Can you work these out from the model? Positions are in its coordinate system, mm. A direction names the side the tool comes from. Coordinates: 2 decimals unless noted, no trailing zeros. Order: outer loops, then holes, each group sorted by start corner. A loop starts at its lowest first (then second) coordinate and runs counter-clockwise, first axis right, second up. Notation, with made-up numbers: (14.5, 24.5) -> (56.5, 24.5) arc R12 ccw to (56.5, 36.5) -> close; hole circle Ø2 at (-8.5, 72). An arc over 180 degrees is marked (long way). Answer as CSV lines item,"result".
from build123d import *

# Parameters (mm, degrees)
F0_R     = 25.527
F0_R_2   = 10.16
F1_DEPTH = 69.85
F0_R_3   = 26.797
F2_DEPTH = 1.27


with BuildPart() as f1:
    # F0 (on Top) → F1 (new body)
    with BuildSketch(Plane.XY):
        Circle(F0_R)
        with BuildLine():
            ThreePointArc((24.223731, 1.27), (24.248681, 0.635218), (24.257, 0))
            ThreePointArc((24.257, 0), (17.595574, -16.69724), (1.27, -24.223731))
            ThreePointArc((1.27, -24.223731), (0.635218, -24.248681), (0, -24.257))
            ThreePointArc((0, -24.257), (-17.152289, -17.152289), (-24.257, 0))
            ThreePointArc((-24.257, 0), (-24.248681, 0.635218), (-24.223731, 1.27))
            ThreePointArc((-24.223731, 1.27), (-16.69724, 17.595574), (0, 24.257))
            ThreePointArc((0, 24.257), (0.635218, 24.248681), (1.27, 24.223731))
            ThreePointArc((1.27, 24.223731), (17.152289, 17.152289), (24.223731, 1.27))
        make_face(mode=Mode.SUBTRACT)
        with BuildLine():
            ThreePointArc((1.27, -11.359225), (8.519419, -7.62), (11.43, 0))
            ThreePointArc((11.43, 0), (11.412293, 0.635985), (11.359225, 1.27))
            ThreePointArc((11.359225, 1.27), (8.082231, 8.082231), (1.27, 11.359225))
            ThreePointArc((1.27, 11.359225), (0.635985, 11.412293), (0, 11.43))
            ThreePointArc((0, 11.43), (-7.62, 8.519419), (-11.359225, 1.27))
            ThreePointArc((-11.359225, 1.27), (-11.412293, 0.635985), (-11.43, 0))
            ThreePointArc((-11.43, 0), (-8.082231, -8.082231), (0, -11.43))
            ThreePointArc((0, -11.43), (0.635985, -11.412293), (1.27, -11.359225))
        make_face()
        Circle(F0_R_2, mode=Mode.SUBTRACT)
        with BuildLine():
            Line((1.27, 11.359225), (1.27, 24.223731))
            ThreePointArc((1.27, 24.223731), (0.635218, 24.248681), (0, 24.257))
            Line((0, 24.257), (0, 11.43))
            ThreePointArc((0, 11.43), (0.635985, 11.412293), (1.27, 11.359225))
        make_face()
        with BuildLine():
            Line((11.43, 0), (24.257, 0))
            ThreePointArc((24.257, 0), (24.248681, 0.635218), (24.223731, 1.27))
            Line((24.223731, 1.27), (11.359225, 1.27))
            ThreePointArc((11.359225, 1.27), (11.412293, 0.635985), (11.43, 0))
        make_face()
        with BuildLine():
            ThreePointArc((0, -24.257), (0.635218, -24.248681), (1.27, -24.223731))
            Line((1.27, -24.223731), (1.27, -11.359225))
            ThreePointArc((1.27, -11.359225), (0.635985, -11.412293), (0, -11.43))
            Line((0, -11.43), (0, -24.257))
        make_face()
        with BuildLine():
            ThreePointArc((-24.223731, 1.27), (-24.248681, 0.635218), (-24.257, 0))
            Line((-24.257, 0), (-11.43, 0))
            ThreePointArc((-11.43, 0), (-11.412293, 0.635985), (-11.359225, 1.27))
            Line((-11.359225, 1.27), (-24.223731, 1.27))
        make_face()
    extrude(amount=F1_DEPTH)

    # F0 (on Top) → F2 (join)
    with BuildSketch(Plane.XY):
        Circle(F0_R_3)
        Circle(F0_R, mode=Mode.SUBTRACT)
    extrude(amount=F2_DEPTH)


solid = f1.part
Q1. Imagine slicing it at D-D (x = 8.5). List the corners of the cut face in (y, z) for me.
Solution:
outline,"(-25.41, 0) -> (-22.72, 0) -> (-22.72, 69.85) -> (-24.07, 69.85) -> (-24.07, 1.27) -> (-25.41, 1.27) -> close; (-7.64, 0) -> (-5.57, 0) -> (-5.57, 69.85) -> (-7.64, 69.85) -> close; (5.57, 0) -> (7.64, 0) -> (7.64, 69.85) -> (5.57, 69.85) -> close; (22.72, 0) -> (25.41, 0) -> (25.41, 1.27) -> (24.07, 1.27) -> (24.07, 69.85) -> (22.72, 69.85) -> close"
Q2. Imagine slicing it at B-B (x = 18). List the corners of the cut face in (y, z) for me.
Solution:
outline,"(-19.85, 0) -> (-16.26, 0) -> (-16.26, 69.85) -> (-18.1, 69.85) -> (-18.1, 1.27) -> (-19.85, 1.27) -> close; (0, 0) -> (1.27, 0) -> (1.27, 69.85) -> (0, 69.85) -> close; (16.26, 0) -> (19.85, 0) -> (19.85, 1.27) -> (18.1, 1.27) -> (18.1, 69.85) -> (16.26, 69.85) -> close"
Q3. Which directions (+Z, -Z, +X, -X, +Y, -Y) give clear straight access to the entire face, cutting with the end or side of a thin tool? Please do faces 5 (the flat face through (1.27, 18, 34)), 6 (the flat face through (-10, 4, 0)).
Solution:
face 5,"+Z, -Z"
face 6,"-Z, +X, -X, +Y, -Y"
Q4. If I drill on line 1 (Y direction, x = -0.5, z = 17.5); line 2 (X direction, y = 13, z = 3); line 3 (X direction, y = 3.5, z = 30), over which ranges is the centre line in solid material (lowest first)?
Solution:
line 1,"-25.52 to -24.25, -11.42 to -10.15, 10.15 to 11.42, 24.25 to 25.52"
line 2,"-21.97 to -20.48, 0 to 1.27, 20.48 to 21.97"
line 3,"-25.29 to -24, -10.88 to -9.54, 9.54 to 10.88, 24 to 25.29"
Q5. We'd pull the mould along X, two halves only. Please class faces 1 (the flat face through (24, -10, 1.27)), 2 (the cylindrical face through (-1.323, 10.074, 34.436)), 3 (the flat face through (0, 18, 34)), 4 (the cylindrical face through (24.348, 7.668, 35.08)): pulls with the +X half, pulls with the -X half, needs draft (parallel to the pull), parting line crosses it, or undercut.
Solution:
face 1,"needs draft"
face 2,"undercut"
face 3,"undercut"
face 4,"parting line crosses it"
Q6. For P1, Ø10, axis at y = 8.5, z = 46.5, coming from the +X side; P2, Ø6, axis at y = -0.5, z = 32, coming from the -X side; P3, Ø12, axis at y = 7.5, z = 49.5, coming from the +X side, each with a flat end and sliding along its axis, tell me the tip position at first contact or that it passes through.
Solution:
P1,"x = 25.29"
P2,"x = -25.53"
P3,"x = 25.48"
Q7. Imagine slicing it at C-C (y = -6). List the corners of the cut face in (x, z) for me, and give its area (3 significant figures).
Solution:
outline,"(-26.12, 0) -> (-23.5, 0) -> (-23.5, 69.85) -> (-24.81, 69.85) -> (-24.81, 1.27) -> (-26.12, 1.27) -> close; (-9.73, 0) -> (-8.2, 0) -> (-8.2, 69.85) -> (-9.73, 69.85) -> close; (8.2, 0) -> (9.73, 0) -> (9.73, 69.85) -> (8.2, 69.85) -> close; (23.5, 0) -> (26.12, 0) -> (26.12, 1.27) -> (24.81, 1.27) -> (24.81, 69.85) -> (23.5, 69.85) -> close"
area,"400 mm2"
Q8. Imagine slicing it at A-A (z = 31.5). List the corners of the cut face in (x, y) for me.
Solution:
outline,"circle Ø51.05 at (0, 0); hole (-24.26, 0) arc R24.26 ccw to (0, -24.26) -> (0, -11.43) arc R11.43 cw to (-11.43, 0) -> close; hole (-24.22, 1.27) -> (-11.36, 1.27) arc R11.43 cw to (0, 11.43) -> (0, 24.26) arc R24.26 ccw to start; hole circle Ø20.32 at (0, 0); hole (1.27, -24.22) arc R24.26 ccw to (24.26, 0) -> (11.43, 0) arc R11.43 cw to (1.27, -11.36) -> close; hole (1.27, 11.36) arc R11.43 cw to (11.36, 1.27) -> (24.22, 1.27) arc R24.26 ccw to (1.27, 24.22) -> close"
